Input: part model. Units: mm. Frame: model coordinates. Face numbers are marked on the shaded views. A direction names the side the tool comes from. Coordinates: 2 decimals unless noted, no trailing zeros. Loops run counter-clockwise (first coordinate to the right, second up) from the corner with the lowest first, then second, coordinate; pieces in that order, holes last. Notation, with made-up numbers: (88.5, 74) - (143.5, 74) arc R20 cw to (143.5, 81) - close; hole circle Ø6 at (66.25, -33.75). An arc over 180 degrees is marked (long way). Use one line per item in the form item = value.
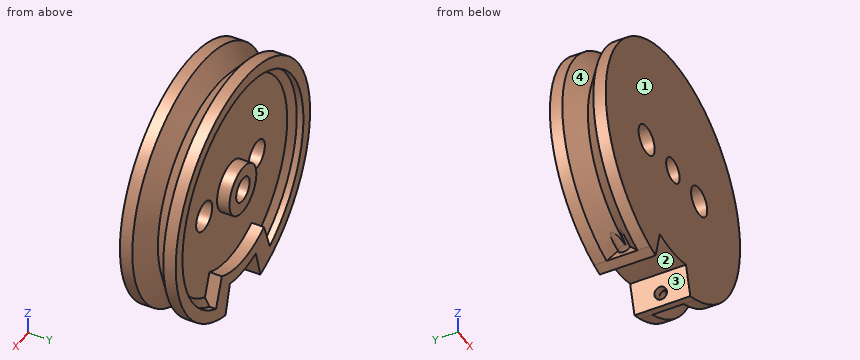
from build123d import *
from build123d.topology import SkipClean

# Parameters (mm, degrees)
CUT_EXTRUDE1_DEPTH       = 15.84082208
SHELL2_START             = 3.968374946
SHELL2_OUTLINE_R         = 2
SHELL2_DEPTH             = 0.531625054
SHELL2_START_2           = 3
SHELL2_3_DEPTH           = 0.968374946
SKETCH6_W                = 2.5
SKETCH6_H                = 4.5
SKETCH6_R                = 0.5
REVOLVE2_ANGLE           = 5
SKETCH9_R                = 0.5
REVOLVE3_ANGLE           = 5
SKETCH13_R               = 0.5
CUT_EXTRUDE3_DEPTH       = 10
CUT_EXTRUDE4_START       = -3
CUT_EXTRUDE4_OUTLINE_R   = 0.5
CUT_EXTRUDE4_DEPTH       = 3
M2_CLEARANCE_HOLE1_D     = 2.4
M2_CLEARANCE_HOLE1_DEPTH = 3.5
M2_CLEARANCE_HOLE1_TIP   = 0.721032743


with BuildPart() as part:
    # Sketch2 → Revolve1 (revolve)
    with BuildSketch(Plane.XY, mode=Mode.PRIVATE) as revolve1_sk:
        Polygon((10, 4.5), (1, 4.5), (1, 0), (10, 0), (10, 1), (8.5, 2.25), (10, 3.5), align=None)
    revolve(revolve1_sk.sketch.rotate(Axis((0, 4.5, 0), (0, -1, 0)), 90), axis=Axis((0, 4.5, 0), (0, -1, 0)))

    # Sketch3 → Cut-Extrude1 (cut, through all)
    with BuildSketch(Plane(origin=(0, 4.5, 0), x_dir=(1, 0, 0), z_dir=(0, 1, 0))):
        with BuildLine():
            Line((-3.420201433, 9.396926208), (-2.565151075, 7.047694656))
            ThreePointArc((-2.565151075, 7.047694656), (0, 7.5), (2.565151075, 7.047694656))
            Line((2.565151075, 7.047694656), (3.420201433, 9.396926208))
            ThreePointArc((3.420201433, 9.396926208), (0, 10), (-3.420201433, 9.396926208))
        make_face()
    extrude(amount=-CUT_EXTRUDE1_DEPTH, mode=Mode.SUBTRACT)

    # Shell2: read off the stored shape, not the designer's step
    # Shell2 outline → Shell2 (cut)
    with BuildSketch(Plane(origin=(0, 0, 0), x_dir=(1, 0, 0), z_dir=(0, 1, 0)).offset(SHELL2_START)):
        with BuildLine():
            Line((-3.136356765, 5.69326499), (-3.998813781, 8.062846169))
            ThreePointArc((-3.998813781, 8.062846169), (0, -9), (3.998813781, 8.062846169))
            Line((3.998813781, 8.062846169), (3.136356765, 5.69326499))
            ThreePointArc((3.136356765, 5.69326499), (0, 6.5), (-3.136356765, 5.69326499))
        make_face()
        Circle(SHELL2_OUTLINE_R, mode=Mode.SUBTRACT)
    extrude(amount=SHELL2_DEPTH, mode=Mode.SUBTRACT)

    # Shell2 2 outline → Shell2 2 (revolve, cut)
    with BuildSketch(Plane.XY):
        Polygon((2, 3.968374946), (2, 3.5), (8.437950065, 3.5), (9, 3.968374946), align=None)
    revolve(axis=Axis((0, 0, 0), (0, 1, 0)), mode=Mode.SUBTRACT)

    # Shell2 3 outline → Shell2 3 (add)
    with BuildSketch(Plane(origin=(0, 0, 0), x_dir=(1, 0, 0), z_dir=(0, 1, 0)).offset(SHELL2_START_2)):
        with BuildLine():
            Line((3.136356765, 5.69326499), (3.998813781, 8.062846169))
            ThreePointArc((3.998813781, 8.062846169), (3.54398789, 8.272856208), (3.07818129, 8.457233587))
            Line((3.07818129, 8.457233587), (2.565151075, 7.047694656))
            ThreePointArc((2.565151075, 7.047694656), (0, 7.5), (-2.565151075, 7.047694656))
            Line((-2.565151075, 7.047694656), (-3.07818129, 8.457233587))
            ThreePointArc((-3.07818129, 8.457233587), (-3.54398789, 8.272856208), (-3.998813781, 8.062846169))
            Line((-3.998813781, 8.062846169), (-3.136356765, 5.69326499))
            ThreePointArc((-3.136356765, 5.69326499), (0, 6.5), (3.136356765, 5.69326499))
        make_face()
    extrude(amount=SHELL2_3_DEPTH)

    # Sketch6 → Revolve2 (revolve)
    with BuildSketch(Plane(origin=(0, 0, 0), x_dir=(-0.3420201433256695, 0, -0.9396926207859082), z_dir=(0.9396926207859082, 0, -0.3420201433256695))):
        with Locations((8.75, 2.25)):
            Rectangle(SKETCH6_W, SKETCH6_H)
        with Locations((9, 2.25)):
            Circle(SKETCH6_R, mode=Mode.SUBTRACT)
    revolve(axis=Axis((0, 0, 0), (0, -1, 0)), revolution_arc=REVOLVE2_ANGLE)

    # Sketch9 → Revolve3 (revolve)
    with SkipClean():  # the faces are left unmerged after this step: merging them gives an invalid solid
        with BuildSketch(Plane(origin=(0, 0, 0), x_dir=(-0.3420201433256693, 0, 0.9396926207859082), z_dir=(-0.9396926207859083, 0, -0.3420201433256693))):
            Polygon((-10, 3.5), (-10, 1), (-10, 0), (-7.5, 0), (-7.5, 4.5), (-10, 4.5), align=None)
            with Locations((-9, 2.25)):
                Circle(SKETCH9_R, mode=Mode.SUBTRACT)
        revolve(axis=Axis((0, 0, 0), (0, 1, 0)), revolution_arc=REVOLVE3_ANGLE)

    # Sketch13 → Cut-Extrude3 (cut)
    with SkipClean():  # the faces are left unmerged after this step: merging them gives an invalid solid
        with BuildSketch(Plane(origin=(0, 0, 0), x_dir=(-0.25881904510252113, 0, 0.9659258262890683), z_dir=(-0.9659258262890683, 0, -0.25881904510252113))):
            with Locations((-9, 2.25)):
                Circle(SKETCH13_R)
        extrude(amount=-CUT_EXTRUDE3_DEPTH, mode=Mode.SUBTRACT)

    # Cut-Extrude4: read off the stored shape, not the designer's step
    # Cut-Extrude4 outline → Cut-Extrude4 (cut)
    with SkipClean():  # the faces are left unmerged after this step: merging them gives an invalid solid
        with BuildSketch(Plane(origin=(0, 0, 0), x_dir=(-0.25881904510252135, 0, -0.9659258262890681), z_dir=(0.9659258262890681, 0, -0.25881904510252135)).offset(CUT_EXTRUDE4_START)):
            with Locations((9, 2.25)):
                Circle(CUT_EXTRUDE4_OUTLINE_R)
        extrude(amount=CUT_EXTRUDE4_DEPTH, mode=Mode.SUBTRACT)

    # M2 Clearance Hole1
    with Locations(Plane(origin=(-3.913029006, 3.5, -0.02653295), x_dir=(0, 0, 1), z_dir=(0, 1, 0))):
        with Locations((0, 0), (0, 7.826058012)):
            Hole(M2_CLEARANCE_HOLE1_D / 2, depth=M2_CLEARANCE_HOLE1_DEPTH)
            with Locations((0, 0, -(M2_CLEARANCE_HOLE1_DEPTH + M2_CLEARANCE_HOLE1_TIP / 2))):  # 118° drill point
                Cone(0, M2_CLEARANCE_HOLE1_D / 2, M2_CLEARANCE_HOLE1_TIP, mode=Mode.SUBTRACT)


solid = part.part
Q1. Ray query, line 1 along X through (y, z) = (4.2, 0); line 2 along Y through (x, z) = (6, -1.25); line 3 along X through (y, z) = (2.9, 0). Return the intervals inside material, ascending. Write a range as [from, to].
Check values:
line_1 = [-10, -9], [-2, -1], [1, 2], [9, 10]
line_2 = [0, 3.5]
line_3 = [-9.28, -5.11], [-2.71, -1], [1, 2.71], [5.11, 9.28]
Q2. Cut plane A-A, the plane x = 0. Return loops of the section in (y, z), then the cut area to 3 significant figures.
Check values:
outline = (0, -7.5) - (4.5, -7.5) - (4.5, -6.5) - (3.5, -6.5) - (3.5, -2) - (4.5, -2) - (4.5, -1) - (0, -1) - close; (0, 1) - (4.5, 1) - (4.5, 2) - (3.5, 2) - (3.5, 8.44) - (3.97, 9) - (4.5, 9) - (4.5, 10) - (3.5, 10) - (2.25, 8.5) - (1, 10) - (0, 10) - close
area = 56.5 mm²
Q3. Pull-direction query (X, two-part tool) for the marked faces 1 and 2; classes: pulls with the +X half, pulls with the -X half, needs draft (parallel to the pull), parting line crosses it, or undercut.
Check values:
face_1 = needs draft
face_2 = undercut
Q4. Set-up query: the marked faces 3, 4 and 5. Return all of +Z, -Z, +X, -X, +Y, -Y with unobstructed straight access to the full face (end or side cutting, diameter ignored); none if empty.
Check values:
face_3 = -Z, +Y, -Y
face_4 = none
face_5 = +Y
Q5. Cut plane B-B, the plane z = 0. Give the number of separate pieces and of enclosed holes in the cut face, then the cut area to 3 significant figures.
Check values:
separate_pieces = 4
enclosed_holes = 0
area = 46.7 mm²
Q6. First-contact query: P1, Ø1, axis at x = -7, y = 2.5, coming from the -Z side; P2, Ø1, axis at x = 4.5, z = 2, coming from the -Y side; P3, Ø2, axis at x = -7, y = 2, coming from the +Z side; P4, Ø1, axis at x = -4.5, y = 3, coming from the -Z side. Flat tips, straight axial feed; report the tip coordinate or a pass-through.
Check values:
P1 = -6.43
P2 = 0
P3 = 7.39
P4 = -8.97
